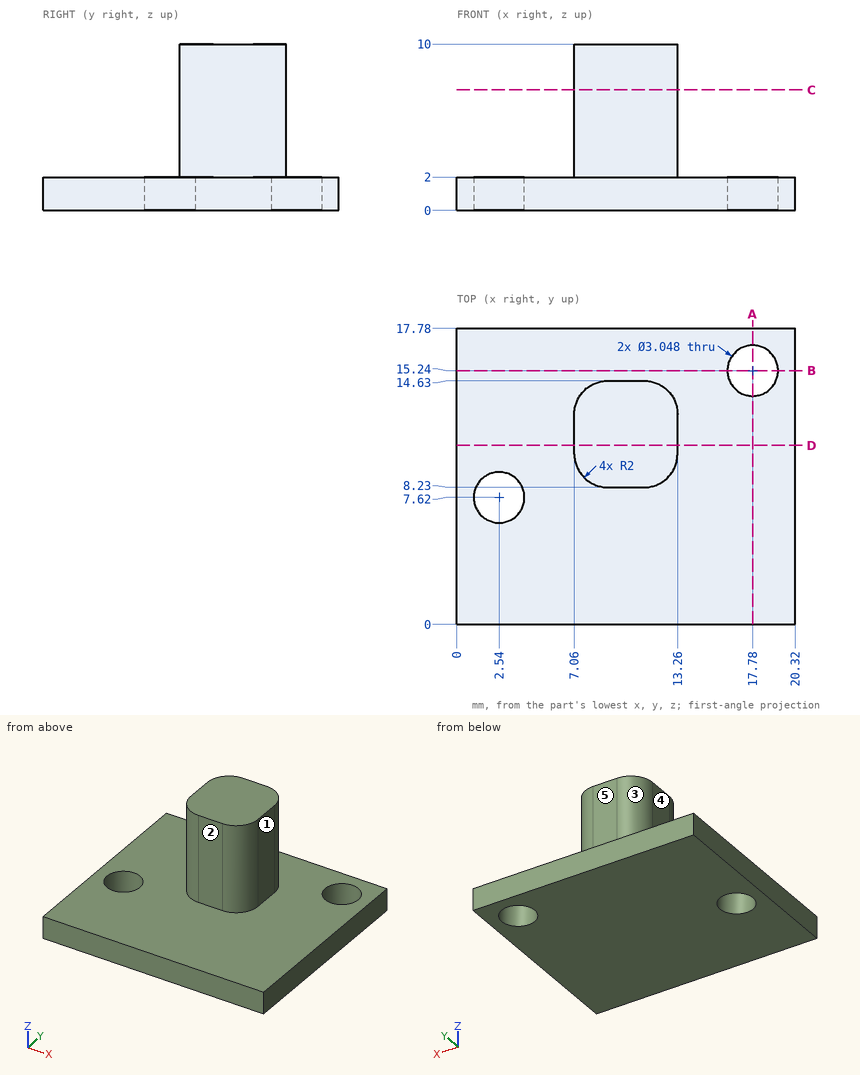
The drawing under review shows one solid part. Ordinate dimensions are in mm from its lowest x, y, z. A direction names the side the tool comes from. Coordinates: 2 decimals unless noted, no trailing zeros. Write each loop counter-clockwise with the first axis right and the second up, starting at its lowest first coordinate (ties: lowest second). Pieces come first, ordered by that corner, then holes.
1) Add section A-A (x = 17.78). Write out the cut boundary in (y, z).
2) To check wall thickness, follow L1, parallel to Y at x = 17.78, z = 0.8; L2, parallel to Y at x = 2.54, z = 1.5; L3, parallel to Z at x = 18.5, y = 13.5. State the ranges of each line that lie inside material, in increasing order.
3) Add section D-D (y = 10.75). Write out the cut boundary in (x, z).
4) Add section B-B (y = 15.24). Write out the cut boundary in (x, z).
5) Machinability: for the marked faces 1, 2, 3, 4 and 5, which of the approach directions +Z, -Z, +X, -X, +Y, -Y give a long, thin tool a straight path to every point of the face, cutting with its end or side? Answer none if there is none.
6) Add section C-C (z = 7.25). Write out the cut boundary in (x, y), plus the area to 3 significant figures.
7) Insertion check: pin 1 (2 mm diameter, centred on x = 2.5, y = 5.5, fed in from -Z); pin 2 (5.5 mm diameter, centred on x = 8, y = 4.5, fed in from +Z); pin 3 (1.8 mm diameter, centred on x = 10.5, z = 7.5, fed in from +Y); pin 4 (1.2 mm diameter, centred on y = 11, z = 7, fed in from +X). Each pin has a flat end and moves straight along its axis. Give the tip position at first contact, or say it passes through.
Check result:
1. outline: (0, 0) - (13.72, 0) - (13.72, 2) - (0, 2) - close; (16.76, 0) - (17.78, 0) - (17.78, 2) - (16.76, 2) - close
2. L1: y = 0 to 13.72, 16.76 to 17.78
2. L2: y = 0 to 6.1, 9.14 to 17.78
2. L3: z = 0 to 2
3. outline: (0, 0) - (20.32, 0) - (20.32, 2) - (13.26, 2) - (13.26, 10) - (7.06, 10) - (7.06, 2) - (0, 2) - close
4. outline: (0, 0) - (16.26, 0) - (16.26, 2) - (0, 2) - close; (19.3, 0) - (20.32, 0) - (20.32, 2) - (19.3, 2) - close
5. face 1: +Z, +X, +Y, -Y
5. face 2: +Z, +X, -X, -Y
5. face 3: +Z, -X, +Y
5. face 4: +Z, -X, +Y, -Y
5. face 5: +Z, +X, -X, +Y
6. outline: (7.06, 10.23) arc R2 ccw to (9.06, 8.23) - (11.26, 8.23) arc R2 ccw to (13.26, 10.23) - (13.26, 12.63) arc R2 ccw to (11.26, 14.63) - (9.06, 14.63) arc R2 ccw to (7.06, 12.63) - close
6. area: 36.2 mm2
7. pin 1: stops at z = 0
7. pin 2: stops at z = 2
7. pin 3: stops at y = 14.63
7. pin 4: stops at x = 13.26
